Can you work these out from the model? Positions are in its coordinate system, mm. Face numbers are marked on the shaded views. A direction names the side the tool comes from. Give positions to 0.01 mm unless a question says otherwise; leave off trailing zeros. Order: outer loops, then holes, each group sorted by start corner. A loop starts at its lowest first (then second) coordinate and runs counter-clockwise, first axis right, second up. Notation, with made-up numbers: (7, 38.25) - (60, 38.25) arc R25 ccw to (60, 58.25) - close; hole circle Ø10 at (0.25, 73.5). An arc over 180 degrees is marked (long way). One line per question, with ' | ' between items.
```python
from build123d import *

# Parameters (mm, degrees)
SKETCH1_R                 = 18
BOSS_EXTRUDE1_DEPTH       = 16
BOSS_EXTRUDE2_DEPTH       = 10
BOSS_EXTRUDE6_DEPTH       = 10
SKETCH5_R                 = 13
CUT_EXTRUDE1_DEPTH        = 13
SKETCH6_R                 = 13
CUT_EXTRUDE2_DEPTH        = 13
SKETCH7_R                 = 8.9
CUT_EXTRUDE3_DEPTH        = 48.882669099
SKETCH8_OUTSIDE_W         = 70.914
SKETCH8_OUTSIDE_H         = 76.54
SKETCH8_OUTSIDE_R         = 18.186533479
CUT_EXTRUDE4_DEPTH        = 5
CUT_EXTRUDE4_DRAFT        = -60
SKETCH9_R                 = 18.186533479
CUT_EXTRUDE5_DEPTH        = 5
CUT_EXTRUDE5_DRAFT        = -60
SKETCH10_W                = 42
SKETCH10_H                = 42
BOSS_EXTRUDE8_DEPTH       = 3
SKETCH11_W                = 37.5
SKETCH11_H                = 37.5
BOSS_EXTRUDE9_DEPTH       = 13
BOSS_EXTRUDE10_REACH      = 71.556
BOSS_EXTRUDE10_END_RADIUS = 18
SKETCH12_W                = 26
SKETCH12_H                = 36


with BuildPart() as part:
    # Sketch1 → Boss-Extrude1 (new, symmetric)
    with BuildSketch(Plane(origin=(0, 0, 0), x_dir=(0, 0, -1), z_dir=(1, 0, 0))):
        Circle(SKETCH1_R)
    extrude(amount=BOSS_EXTRUDE1_DEPTH, both=True)

    # Sketch2 → Boss-Extrude2 (add)
    with BuildSketch(Plane(origin=(16, 0, 0), x_dir=(0, 0, -1), z_dir=(1, 0, 0))):
        Polygon((0, 21), (-18.186533479, 10.5), (-18.186533479, -10.5), (0, -21), (18.186533479, -10.5), (18.186533479, 10.5), align=None)
    extrude(amount=BOSS_EXTRUDE2_DEPTH)

    # Sketch4 → Boss-Extrude6 (add)
    with BuildSketch(Plane.ZY.offset(16)):
        Polygon((18.186533479, 10.5), (0, 21), (-18.186533479, 10.5), (-18.186533479, -10.5), (0, -21), (18.186533479, -10.5), align=None)
    extrude(amount=BOSS_EXTRUDE6_DEPTH)

    # Sketch5 → Cut-Extrude1 (cut)
    with BuildSketch(Plane.ZY.offset(26)):
        Circle(SKETCH5_R)
    extrude(amount=-CUT_EXTRUDE1_DEPTH, mode=Mode.SUBTRACT)

    # Sketch6 → Cut-Extrude2 (cut)
    with BuildSketch(Plane(origin=(26, 0, 0), x_dir=(0, 0, -1), z_dir=(1, 0, 0))):
        with Locations(Location((0, 0, 0), (0, 0, 180))):
            Circle(SKETCH6_R)
    extrude(amount=-CUT_EXTRUDE2_DEPTH, mode=Mode.SUBTRACT)

    # Sketch7 → Cut-Extrude3 (cut, through all)
    with BuildSketch(Plane(origin=(13, 0, 0), x_dir=(0, 0, -1), z_dir=(1, 0, 0))):
        Circle(SKETCH7_R)
    extrude(amount=-CUT_EXTRUDE3_DEPTH, mode=Mode.SUBTRACT)


with BuildPart() as cut_extrude4_tool:
    # Sketch8 outside → Cut-Extrude4 (with draft: the straight prism first)
    with BuildSketch(Plane(origin=(26, 0, 0), x_dir=(0, 0, -1), z_dir=(1, 0, 0))):
        Rectangle(SKETCH8_OUTSIDE_W, SKETCH8_OUTSIDE_H)
        Circle(SKETCH8_OUTSIDE_R, mode=Mode.SUBTRACT)
    extrude(amount=-CUT_EXTRUDE4_DEPTH)
    # Cut-Extrude4: the draft: its side faces are tilted about the plane it starts from
    cut_extrude4_sides = [cut_extrude4_tool.faces().sort_by_distance(p)[0] for p in [
        (23.5, -38.27, 0),
        (23.5, 0, -35.457),
        (23.5, 38.27, 0),
        (23.5, 0, 35.457),
        (23.5, 0, 18.186533479),
    ]]
    draft(cut_extrude4_sides, Plane(origin=(26, 0, 0), x_dir=(0, 0, -1), z_dir=(1, 0, 0)), CUT_EXTRUDE4_DRAFT)


with BuildPart() as part_1:
    add(part.part)

    # Cut-Extrude4: cut by cut_extrude4_tool
    add(cut_extrude4_tool.part, mode=Mode.SUBTRACT)


with BuildPart() as cut_extrude5_tool:
    # Sketch9 → Cut-Extrude5 (with draft: the straight prism first)
    with BuildSketch(Plane.ZY.offset(26)):
        Circle(SKETCH9_R)
    extrude(amount=-CUT_EXTRUDE5_DEPTH)
    # Cut-Extrude5: the draft: its side faces are tilted about the plane it starts from
    cut_extrude5_sides = [cut_extrude5_tool.faces().sort_by_distance(p)[0] for p in [
        (-23.5, 0, -18.186533479),
    ]]
    draft(cut_extrude5_sides, Plane.ZY.offset(26), CUT_EXTRUDE5_DRAFT)


with BuildPart() as part_2:
    add(part_1.part)

    # Cut-Extrude5: cut by cut_extrude5_tool
    add(cut_extrude5_tool.part, mode=Mode.SUBTRACT)



with BuildPart() as body_2:
    # Sketch10 → Boss-Extrude8 (new body)
    with BuildSketch(Plane(origin=(0, 40, 0), x_dir=(1, 0, 0), z_dir=(0, 1, 0))):
        Rectangle(SKETCH10_W, SKETCH10_H)
    extrude(amount=-BOSS_EXTRUDE8_DEPTH)

    # Sketch11 → Boss-Extrude9 (add)
    with BuildSketch(Plane(origin=(0, 40, 0), x_dir=(1, 0, 0), z_dir=(0, 1, 0))):
        Rectangle(SKETCH11_W, SKETCH11_H)
    extrude(amount=-BOSS_EXTRUDE9_DEPTH)


with BuildPart() as part_3:
    add(part_2.part)

    add(body_2.part)  # Boss-Extrude10 merges body 2
    # Boss-Extrude10: up to this cylinder (the profile starts outside it)
    boss_extrude10_end = Plane(origin=(0, 0, 0), z_dir=(-1, 0, 0)) * Cylinder(BOSS_EXTRUDE10_END_RADIUS, 180.112, mode=Mode.PRIVATE)
    # Sketch12 → Boss-Extrude10 (add, up to the surface)
    with BuildSketch(Plane(origin=(0, 40, 0), x_dir=(1, 0, 0), z_dir=(0, 1, 0)), mode=Mode.PRIVATE) as boss_extrude10_sk1:
        Rectangle(SKETCH12_W, SKETCH12_H)
    boss_extrude10_tool1 = extrude(boss_extrude10_sk1.sketch, amount=-BOSS_EXTRUDE10_REACH, mode=Mode.PRIVATE) - boss_extrude10_end
    add(boss_extrude10_tool1.solids().sort_by_distance((0, 40, 0))[0])

    # Sketch13 → Cut-Revolve1 (revolve, cut)
    with BuildSketch(Plane.XY, mode=Mode.PRIVATE) as cut_revolve1_sk:
        Polygon((0, 40), (0, -9.9), (7, -9.9), (9, 16.1), (10, 16.1), (10, 30.604253251), (18, 30.604253251), (18, 40), align=None)
    revolve(cut_revolve1_sk.sketch.rotate(Axis((0, 40, 0), (0, -1, 0)), 180), axis=Axis((0, 40, 0), (0, -1, 0)), mode=Mode.SUBTRACT)


solid = part_3.part
```
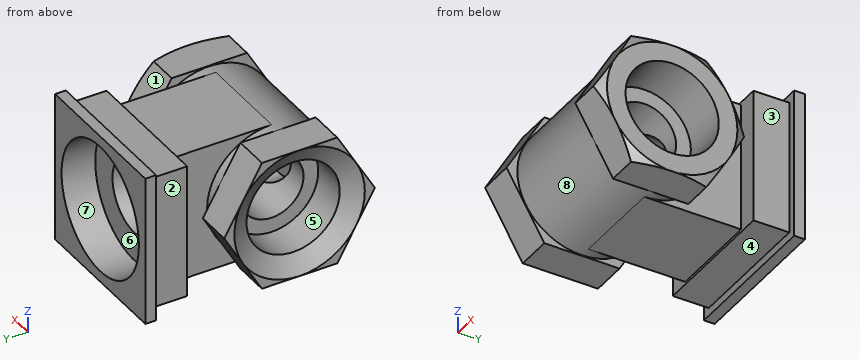
(1) If I drill on line 1 (Y direction, x = 20.5, z = 0); line 2 (Z direction, x = -18.25, y = 0); line 3 (Z direction, x = 0, y = 33), over which ranges is the centre line in solid material (lowest first)?
Answer below:
line 1: -21 to -13, 13 to 21, 37 to 40 | line 2: -18.19 to -13, 13 to 18.19 | line 3: -18.75 to -18, 18 to 18.75
(2) If we mould it in two halves opening along Y, with no side actions, what happens to the marked faces 6, 7 and 8? For each: released by +Y, released by -Y, zero draft, split by the parting line, or undercut.
Answer below:
face 6: released by +Y | face 7: zero draft | face 8: undercut
(3) Imagine slicing it at A-A (x = 17). List the corners of the cut face in (y, z) for me, and give its area (3 significant figures).
Answer below:
outline: (-21, 0) - (-10.5, -18.19) - (10.5, -18.19) - (21, 0) - (10.5, 18.19) - (-10.5, 18.19) - close; (27, -18.75) - (37, -18.75) - (37, -21) - (40, -21) - (40, -5.92) - (30.6, -5.92) - (30.6, 5.92) - (40, 5.92) - (40, 21) - (37, 21) - (37, 18.75) - (27, 18.75) - close; hole circle Ø26 at (0, 0) | area: 1,000 mm^2
(4) Imagine slicing it at C-C (z = -3.5). Count the separate pieces of the cut face and the enclosed holes in it, and give its area (3 significant figures).
Answer below:
separate pieces: 3 | enclosed holes: 0 | area: 789 mm^2
(5) On a 3-axis mill with a long thin cutter (end or side, diameter ignored), from which of +Z, -Z, +X, -X, +Y, -Y can I reach the whole of each face in a straight line? I mean the marked faces 1, 2, 3, 4 and 5. Say none if no direction works.
Answer below:
face 1: +Z, +X | face 2: +Z, -Z, -X | face 3: +Z, -Z, +X | face 4: -Z, +X, -X, -Y | face 5: -X
(6) Will these pins go through, and if not, where does the flat tip stop? pin 1 (8 mm diameter, centred on x = -19, y = -2.5, fed in from +Z); pin 2 (5 mm diameter, centred on x = -21, y = 0, fed in from -Z); pin 3 (11 mm diameter, centred on y = 32.5, z = 3, fed in from -X).
Answer below:
pin 1: z = 18.19 | pin 2: z = -18.19 | pin 3: x = -21
(7) Imagine slicing it at B-B (x = 0). List the corners of the cut face in (y, z) for me, and give its area (3 significant figures).
Answer below:
outline: (-9.9, -7) - (-9.9, 7) - (-4.98, 7.38) arc R8.9 cw to (3.79, 8.05) - (16.1, 9) - (16.1, 10) - (30.6, 10) - (30.6, 18) - (40, 18) - (40, 21) - (37, 21) - (37, 18.75) - (27, 18.75) - (27, 18) - (0, 18) arc R18 ccw to (0, -18) - (27, -18) - (27, -18.75) - (37, -18.75) - (37, -21) - (40, -21) - (40, -18) - (30.6, -18) - (30.6, -10) - (16.1, -10) - (16.1, -9) - (3.79, -8.05) arc R8.9 cw to (-4.98, -7.38) - close | area: 924 mm^2
